Model file for the job. Use its own axes, mm. Face numbers are marked on the shaded views. A direction names the side the tool comes from. Give positions to 0.01 mm unless a question says otherwise; leave off trailing zeros. Write each loop counter-clockwise with the first axis right and the second up, starting at its lowest first coordinate (ties: lowest second). Pieces come first, ordered by that corner, then holes. Notation, with made-up numbers: (64.5, 31.5) - (108.5, 31.5) arc R22 ccw to (108.5, 61.5) - close; hole circle Ø7 at (51, -14.5). An arc over 180 degrees is marked (long way). One line per item, written item: value. Start each with the question number.
(1) Drop flat-ended pins along their axis: P1, Ø1.5, axis at x = -2.5, z = -9, coming from the +Y side; P2, Ø2.5, axis at x = 0, y = 14.5, coming from the +Z side; P3, Ø1, axis at x = 1, z = 7, coming from the +Y side. Give the stop position or say it passes through.
(2) Probe L1, parallel to Z at x = -1.25, y = 2; L2, parallel to Y at x = -1, z = 0; L3, parallel to Z at x = -3.25, y = 1. List the from-to ranges inside material, lowest first.
(3) Cut at A-A, the plane z = 0.5. List the corners of the cut face in (x, y).
(4) Mould opens along Z. For the marked faces 4, 5 and 6 say: pulls with the +Z half, pulls with the -Z half, needs draft (parallel to the pull), parting line crosses it, or undercut.
(5) Cut at D-D, the plane y = 10.5. List the corners of the cut face in (x, z).
(6) 3-axis set-ups, long thin cutter, end or side, ignore diameter. For the marked faces 1, 2 and 3: which of +Z, -Z, +X, -X, +Y, -Y reach the whole face in a straight line?
(7) Cut at C-C, the plane y = 1. List the corners of the cut face in (x, z), and give its area (3 significant figures).
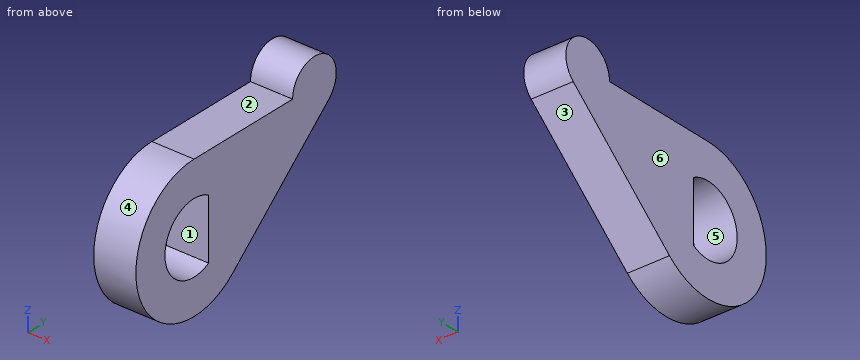
from build123d import *

# Parameters (mm, degrees)
BOSS_EXTRUDE1_DEPTH = 3.81


with BuildPart() as part:
    # Sketch1 → Boss-Extrude1 (new, symmetric)
    with BuildSketch(Plane(origin=(0, 0, 0), x_dir=(0, 0, -1), z_dir=(1, 0, 0))):
        with BuildLine():
            Line((-12.7, 0), (-12.7, 21.524540775))
            ThreePointArc((-12.7, 21.524540775), (-17.043342208, 28.240700088), (-9.136572828, 29.446691553))
            Line((-9.136572828, 29.446691553), (9.502472459, 8.425735408))
            ThreePointArc((9.502472459, 8.425735408), (4.506029281, -11.873739938), (-12.7, 0))
        make_face()
        with BuildLine():
            Line((-5.4991, 3.175279388), (5.4991, 3.175279388))
            ThreePointArc((5.4991, 3.175279388), (0, -6.35), (-5.4991, 3.175279388))
        make_face(mode=Mode.SUBTRACT)
    extrude(amount=BOSS_EXTRUDE1_DEPTH, both=True)


solid = part.part
Answers follow:
1. P1: stops at y = 9.84
1. P2: stops at z = 12.7
1. P3: stops at y = 27.6
2. L1: z = -12.54 to -6.03, 6.03 to 12.7
2. L2: y = -12.7 to -6.35, 3.18 to 19.14
2. L3: z = -12.66 to -6.27, 6.27 to 12.7
3. outline: (-3.81, -12.69) - (3.81, -12.69) - (3.81, -6.33) - (-3.81, -6.33) - close; (-3.81, 3.18) - (3.81, 3.18) - (3.81, 19.71) - (-3.81, 19.71) - close
4. face 4: parting line crosses it
4. face 5: undercut
4. face 6: needs draft
5. outline: (-3.81, -7.66) - (3.81, -7.66) - (3.81, 12.7) - (-3.81, 12.7) - close
6. face 1: +X, -X
6. face 2: +Z, +X, -X, -Y
6. face 3: -Z, +X, -X, +Y
7. outline: (-3.81, -12.66) - (3.81, -12.66) - (3.81, -6.27) - (-3.81, -6.27) - close; (-3.81, 6.27) - (3.81, 6.27) - (3.81, 12.7) - (-3.81, 12.7) - close
7. area: 97.7 mm²
